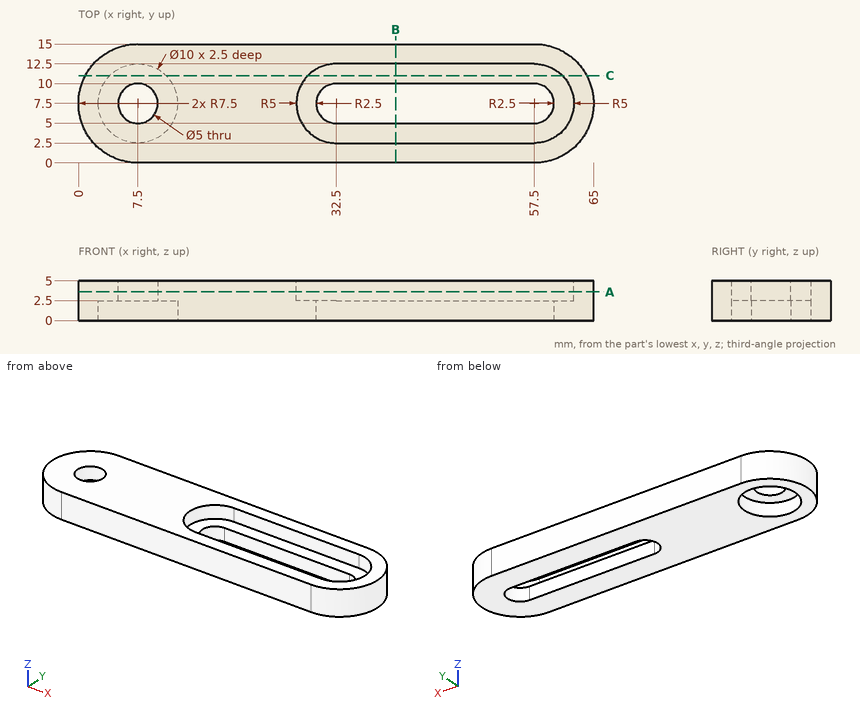
Job drawing, mm, ordinate dimensions from the low corner. One solid piece. Round coordinates to 2 decimals unless told otherwise and drop trailing zeros. Order: outer loops, then holes, each group sorted by start corner. A loop starts at its lowest first (then second) coordinate and runs counter-clockwise, first axis right, second up. Notation, with made-up numbers: (82, -18.75) - (127, -18.75) arc R14 ccw to (127, 6.25) - close; hole circle Ø5 at (88.25, -37.75). An arc over 180 degrees is marked (long way). Use CSV: the item, a comma, the result in double quotes. Start each with the question number.
1) Saw through at B-B (x = 40). List the corners of the cut face in (y, z), and give its area (3 significant figures).
2) Saw through at C-C (y = 11). List the corners of the cut face in (x, z).
3) Wall check: L1, parallel to Y at x = 36, z = 1.4; L2, parallel to Y at x = 33, z = 4.7; L3, parallel to X at y = 8, z = 4.5. Give the ranges that are in metal, low to high. Write a range as [from, to].
4) Saw through at A-A (z = 3.6). List the corners of the cut face in (x, y).
5) Pin check, flat tips, straight feed: pin 1 Ø8 at (x, y) = (37.5, 7) entering from +Z; pin 2 Ø1.5 at (y, z) = (4, 3) entering from -X; pin 3 Ø2 at (y, z) = (4.5, 3.5) entering from +X. Stop position of each tip, or through.
Values follow:
1,outline,"(0, 0) - (5, 0) - (5, 2.5) - (2.5, 2.5) - (2.5, 5) - (0, 5) - close; (10, 0) - (15, 0) - (15, 5) - (12.5, 5) - (12.5, 2.5) - (10, 2.5) - close"
1,area,"37.5 mm2"
2,outline,"(0.87, 0) - (3.93, 0) - (3.93, 2.5) - (11.07, 2.5) - (11.07, 0) - (64.13, 0) - (64.13, 5) - (61.07, 5) - (61.07, 2.5) - (28.93, 2.5) - (28.93, 5) - (0.87, 5) - close"
3,L1,"y = [0, 5], [10, 15]"
3,L2,"y = [0, 2.5], [12.5, 15]"
3,L3,"x = [0.02, 5.05], [9.95, 27.53], [62.47, 64.98]"
4,outline,"(7.5, 0) - (57.5, 0) arc R7.5 ccw to (57.5, 15) - (7.5, 15) arc R7.5 ccw to start; hole circle Ø5 at (7.5, 7.5); hole (32.5, 2.5) - (57.5, 2.5) arc R5 ccw to (57.5, 12.5) - (32.5, 12.5) arc R5 ccw to start"
5,pin 1,"stops at z = 2.5"
5,pin 2,"stops at x = 0.52"
5,pin 3,"stops at x = 64.73"
